For this review, take the finished solid that the model builds, in its own axes (mm). A direction names the side the tool comes from. Round coordinates to 2 decimals unless told otherwise and drop trailing zeros. Write each loop counter-clockwise with the first axis right and the second up, starting at its lowest first coordinate (ties: lowest second). Pieces come first, ordered by that corner, then holes. Notation, with made-up numbers: (63.25, 22.25) -> (102.25, 22.25) arc R23 ccw to (102.25, 42.25) -> close; hole circle Ø6 at (25.5, 31). An arc over 180 degrees is marked (long way). Answer in a Markdown table with one row per item. Add a question column.
```python
from build123d import *

# Parameters (mm, degrees)
SKETCH1_W                = 40
SKETCH1_H                = 40
SKETCH1_H_2              = 10
SKETCH1_W_2              = 903
SKETCH1_H_3              = 2060
BOSS_EXTRUDE1_DEPTH      = 65
BOSS_EXTRUDE2_DEPTH      = 350
BOSS_EXTRUDE2_DEPTH_BACK = 50
SKETCH1_3_W              = 943
SKETCH1_3_H              = 80
SKETCH1_4_W              = 40
SKETCH1_4_H              = 40
BOSS_EXTRUDE3_DEPTH      = 240
BOSS_EXTRUDE4_DEPTH      = 30
BOSS_EXTRUDE5_DEPTH      = 30
SKETCH5_W                = 30
SKETCH5_H                = 30
CUT_EXTRUDE1_DEPTH       = 200
BOSS_EXTRUDE6_DEPTH      = 30
BOSS_EXTRUDE7_START      = -30
BOSS_EXTRUDE7_DEPTH      = 30
BOSS_EXTRUDE8_DEPTH      = 20
BOSS_EXTRUDE8_DEPTH_BACK = 20
SKETCH8_W                = 743
SKETCH8_H                = 450
BOSS_EXTRUDE9_DEPTH      = 130
SKETCH9_W                = 50
SKETCH9_H                = 50
BOSS_EXTRUDE11_DEPTH     = 750
SKETCH9_3_W              = 50
SKETCH9_3_H              = 50
BOSS_EXTRUDE12_DEPTH     = 1170
SKETCH10_W               = 50
SKETCH10_H               = 50
BOSS_EXTRUDE13_DEPTH     = 85
BOSS_EXTRUDE14_DEPTH     = 20
BOSS_EXTRUDE15_DEPTH     = 20
SKETCH14_W               = 943
SKETCH14_H               = 30
BOSS_EXTRUDE16_DEPTH     = 105


with BuildPart() as part:
    # Sketch1 → Boss-Extrude1 (new body)
    with BuildSketch(Plane(origin=(0, 0, 0), x_dir=(1, 0, 0), z_dir=(0, 1, 0))):
        with Locations((-431.5, 20)):
            Rectangle(SKETCH1_W, SKETCH1_H)
        Polygon((-411.5, 50), (-411.5, 40), (-411.5, 0), (411.5, 0), (411.5, 40), (411.5, 50), align=None)
        with Locations((-431.5, 45)):
            Rectangle(SKETCH1_W, SKETCH1_H_2)
        Polygon((-451.5, 0), (-451.5, 40), (-451.5, 50), (-451.5, 60), (-471.5, 60), (-471.5, -20), (471.5, -20), (471.5, 60), (451.5, 60), (451.5, 50), (451.5, 40), (451.5, 0), (411.5, 0), (-411.5, 0), align=None)
        Polygon((-451.5, 50), (-411.5, 50), (411.5, 50), (451.5, 50), (451.5, 60), (-451.5, 60), align=None)
        with Locations((431.5, 20)):
            Rectangle(SKETCH1_W, SKETCH1_H)
        with Locations((431.5, 45)):
            Rectangle(SKETCH1_W, SKETCH1_H_2)
        with Locations((0, 1090)):
            Rectangle(SKETCH1_W_2, SKETCH1_H_3)
        Polygon((-471.5, 2120), (-451.5, 2120), (-451.5, 2130), (-451.5, 2140), (-451.5, 2180), (-411.5, 2180), (411.5, 2180), (451.5, 2180), (451.5, 2140), (451.5, 2130), (451.5, 2120), (471.5, 2120), (471.5, 2200), (-471.5, 2200), align=None)
        Polygon((-451.5, 2130), (-451.5, 2120), (451.5, 2120), (451.5, 2130), (411.5, 2130), (-411.5, 2130), align=None)
        with Locations((-431.5, 2135)):
            Rectangle(SKETCH1_W, SKETCH1_H_2)
        with Locations((-431.5, 2160)):
            Rectangle(SKETCH1_W, SKETCH1_H)
        Polygon((-411.5, 2140), (-411.5, 2130), (411.5, 2130), (411.5, 2140), (411.5, 2180), (-411.5, 2180), align=None)
        with Locations((431.5, 2135)):
            Rectangle(SKETCH1_W, SKETCH1_H_2)
        with Locations((431.5, 2160)):
            Rectangle(SKETCH1_W, SKETCH1_H)
    extrude(amount=-BOSS_EXTRUDE1_DEPTH)

    # Sketch1<3> → Boss-Extrude2 (add, two sides: drawn at the far end of the back side and taken through both)
    with BuildSketch(Plane(origin=(0, 0, 0), x_dir=(1, 0, 0), z_dir=(0, 1, 0)).offset(-BOSS_EXTRUDE2_DEPTH_BACK)):
        with Locations((0, 2160)):
            Rectangle(SKETCH1_3_W, SKETCH1_3_H)
        with Locations((0, 20)):
            Rectangle(SKETCH1_3_W, SKETCH1_3_H)
    extrude(amount=BOSS_EXTRUDE2_DEPTH + BOSS_EXTRUDE2_DEPTH_BACK)

    # Sketch1<4> → Boss-Extrude3 (add)
    with BuildSketch(Plane(origin=(0, 0, 0), x_dir=(1, 0, 0), z_dir=(0, 1, 0))):
        with Locations((431.5, 2160)):
            Rectangle(SKETCH1_4_W, SKETCH1_4_H)
        with Locations((-431.5, 2160)):
            Rectangle(SKETCH1_4_W, SKETCH1_4_H)
        with Locations((-431.5, 20)):
            Rectangle(SKETCH1_4_W, SKETCH1_4_H)
        with Locations((431.5, 20)):
            Rectangle(SKETCH1_4_W, SKETCH1_4_H)
    extrude(amount=-BOSS_EXTRUDE3_DEPTH)

    # Sketch3 → Boss-Extrude4 (add)
    with BuildSketch(Plane(origin=(451.5, 0, 0), x_dir=(0, 0, -1), z_dir=(1, 0, 0))):
        Polygon((40, -65), (40, -225), (110, -225), (150, -65), align=None)
        Polygon((2140, -65), (2030, -65), (2070, -225), (2140, -225), align=None)
    extrude(amount=-BOSS_EXTRUDE4_DEPTH)

    # Sketch4 → Boss-Extrude5 (add)
    with BuildSketch(Plane(origin=(-451.5, 0, -45.75), x_dir=(0, 0, -1), z_dir=(1, 0, 0))):
        Polygon((2024.25, -225), (2094.25, -225), (2094.25, -65), (1984.25, -65), align=None)
        Polygon((64.25, -225), (104.25, -65), (-5.75, -65), (-5.75, -225), align=None)
    extrude(amount=BOSS_EXTRUDE5_DEPTH)

    # Sketch5 → Cut-Extrude1 (cut)
    with BuildSketch(Plane.XZ.offset(240)):
        with Locations((-431.5, -2160)):
            Rectangle(SKETCH5_W, SKETCH5_H)
        with Locations((431.5, -2160)):
            Rectangle(SKETCH5_W, SKETCH5_H)
        with Locations((431.5, -20)):
            Rectangle(SKETCH5_W, SKETCH5_H)
        with Locations((-431.5, -20)):
            Rectangle(SKETCH5_W, SKETCH5_H)
    extrude(amount=-CUT_EXTRUDE1_DEPTH, mode=Mode.SUBTRACT)

    # Sketch6 → Boss-Extrude6 (add)
    with BuildSketch(Plane.XY.offset(20)):
        with BuildLine():
            Line((130, -65), (-130, -65))
            ThreePointArc((-130, -65), (0, -195), (130, -65))
        make_face()
    extrude(amount=-BOSS_EXTRUDE6_DEPTH)

    # Sketch7 → Boss-Extrude7 (add)
    with BuildSketch(Plane(origin=(0, 0, -2200), x_dir=(-1, 0, 0), z_dir=(0, 0, -1)).offset(BOSS_EXTRUDE7_START)):
        with BuildLine():
            Line((130, -65), (-130, -65))
            ThreePointArc((-130, -65), (0, -195), (130, -65))
        make_face()
    extrude(amount=BOSS_EXTRUDE7_DEPTH)

    # 3DSketch1 → Boss-Extrude8 (add, two sides: drawn at the far end of the back side and taken through both)
    with BuildSketch(Plane(origin=(0, -195, -10), x_dir=(0, 0.018515344006020947, -0.9998285763251313), z_dir=(1, 0, 0)).offset(-BOSS_EXTRUDE8_DEPTH_BACK)):
        Polygon((0, 0), (0.74061376, 39.993143053), (2160.370338623, 0), (2159.629724862, -39.993143053), align=None)
    extrude(amount=BOSS_EXTRUDE8_DEPTH + BOSS_EXTRUDE8_DEPTH_BACK)

    # Sketch8 → Boss-Extrude9 (add)
    with BuildSketch(Plane.XZ.offset(65)):
        with Locations((0, -205)):
            Rectangle(SKETCH8_W, SKETCH8_H)
    extrude(amount=BOSS_EXTRUDE9_DEPTH)

    # Sketch9 → Boss-Extrude11 (add)
    with BuildSketch(Plane(origin=(0, 0, -430), x_dir=(-1, 0, 0), z_dir=(0, 0, -1))):
        with Locations((-346.5, -75)):
            Rectangle(SKETCH9_W, SKETCH9_H)
    extrude(amount=BOSS_EXTRUDE11_DEPTH)

    # Sketch9<3> → Boss-Extrude12 (add)
    with BuildSketch(Plane(origin=(0, 0, -430), x_dir=(-1, 0, 0), z_dir=(0, 0, -1))):
        with Locations((346.5, -125)):
            Rectangle(SKETCH9_3_W, SKETCH9_3_H)
    extrude(amount=BOSS_EXTRUDE12_DEPTH)

    # Sketch10 → Boss-Extrude13 (add)
    with BuildSketch(Plane.XZ.offset(150)):
        with Locations((-346.5, -1575)):
            Rectangle(SKETCH10_W, SKETCH10_H)
    extrude(amount=-BOSS_EXTRUDE13_DEPTH)

    # Sketch12 → Boss-Extrude14 (add)
    with BuildSketch(Plane.ZY.offset(451.5)):
        Polygon((-60, 0), (-2120, 0), (-2120, -65), (-2180, -65), (-2180, -240), (-2140, -240), (-2140, -225), (-2070, -225), (-2030, -65), (-150, -65), (-110, -225), (-40, -225), (-40, -240), (0, -240), (0, -65), (-60, -65), align=None)
    extrude(amount=BOSS_EXTRUDE14_DEPTH)

    # Sketch13 → Boss-Extrude15 (add)
    with BuildSketch(Plane(origin=(451.5, 0, 0), x_dir=(0, 0, -1), z_dir=(1, 0, 0))):
        Polygon((2120, 0), (60, 0), (60, -65), (0, -65), (0, -240), (40, -240), (40, -225), (110, -225), (150, -65), (2030, -65), (2070, -225), (2140, -225), (2140, -240), (2180, -240), (2180, -65), (2120, -65), align=None)
    extrude(amount=BOSS_EXTRUDE15_DEPTH)

    # Sketch14 → Boss-Extrude16 (add)
    with BuildSketch(Plane.XZ.offset(65)):
        with Locations((0, -395)):
            Rectangle(SKETCH14_W, SKETCH14_H)
    extrude(amount=BOSS_EXTRUDE16_DEPTH)


solid = part.part
```
1. For L1, parallel to Z at x = 165, y = 294; L2, parallel to Z at x = 35.5, y = -125; L3, parallel to Y at x = 306.5, z = -1394.5, list the stretches that pass through material, from the lowest coordinate up. Write a range as [from, to].
2. We need section A-A (y = 260.5). Write out the cut boundary in (x, z).
3. Tool access review of faces 3 (the flat face through (411.5, -151, -20)), 4 (the flat face through (-7, 173, -60)), 5 (the flat face through (-346, -107, -1600)), 6 (the flat face through (-421.5, -144, -2096)): name each direction out of +Z, -Z, +X, -X, +Y, -Y from which nothing blocks a thin tool from reaching the whole face with its end or side.
4. We need section C-C (x = 154). Write out the cut boundary in (y, z).
5. We need section B-B (z = -882.5). Write out the cut boundary in (x, y), plus the area to 3 significant figures.
6. Clearance check with flat-ended pins moving along their axes: pin 1 Ø9 at (x, y) = (427.5, -110) entering from -Z; pin 2 Ø1.5 at (x, z) = (82, -1232.5) entering from +Y; pin 3 Ø1 at (x, z) = (-84, -1661.5) entering from -Y. State where each tip first meets the part, or that it passes through.
7. The part is to be moulded in two halves that separate along X. For faces 1 (the flat face through (2, -114, -2170)), 2 (the flat face through (347, -100, -800)), say which applies: pulls with the +X half, pulls with the -X half, needs draft (parallel to the pull), parting line crosses it, or undercut.
Response:
| question | item | result |
|---|---|---|
| 1 | L1 | [-2200, -2120], [-60, 20] |
| 1 | L2 | [-2200, -2170], [-430, 20] |
| 1 | L3 | [-65, 0] |
| 2 | outline | (-471.5, -2200) -> (471.5, -2200) -> (471.5, -2120) -> (-471.5, -2120) -> close; (-471.5, -60) -> (471.5, -60) -> (471.5, 20) -> (-471.5, 20) -> close |
| 3 | face 3 | +Z, -Y |
| 3 | face 4 | +X, -X, +Y |
| 3 | face 5 | -Z, +X, -X, -Y |
| 3 | face 6 | -Y |
| 4 | outline | (-195, -430) -> (-65, -430) -> (-65, -2200) -> (350, -2200) -> (350, -2120) -> (0, -2120) -> (0, -60) -> (350, -60) -> (350, 20) -> (-195, 20) -> close |
| 5 | outline | (-471.5, -65) -> (321.5, -65) -> (321.5, -100) -> (371.5, -100) -> (371.5, -65) -> (471.5, -65) -> (471.5, 0) -> (-471.5, 0) -> close; (-371.5, -150) -> (-321.5, -150) -> (-321.5, -100) -> (-371.5, -100) -> close; (-20, -195) -> (20, -195) -> (20, -155) -> (-20, -155) -> close |
| 5 | area | 67,100 mm2 |
| 6 | pin 1 | z = -2180 |
| 6 | pin 2 | y = 0 |
| 6 | pin 3 | y = -65 |
| 7 | face 1 | undercut |
| 7 | face 2 | needs draft |
